Autodesk Fusion 360 part; units mm, degrees
sketch "Sketch1" plane through (0, 0, 0) normal (0, 0, 1) x (1, 0, 0)
  circle A0 centre (0, 0) radius 15 construction
  circle A1 centre (0, 15) radius 1.7
  circle A2 centre (-15, 0) radius 1.7
  circle A3 centre (0, -15) radius 1.7
  circle A4 centre (15, 0) radius 1.7
  circle A5 centre (0, 0) radius 25
  circle A6 centre (0, 25) radius 1.5 construction
  circle A7 centre (-25, 0) radius 1.5 construction
  circle A8 centre (0, -25) radius 1.5 construction
  circle A9 centre (25, 0) radius 1.5 construction
  circle A10 centre (0, 0) radius 31.5
  circle A11 centre (0, 0) radius 25 construction
  dimension "d426" = 30
  dimension "d427" = 3.4
  dimension "d429" = 360
  dimension "d430" = 50
  dimension "d432" = 3
  dimension "d442" = 63
  dimension "d443" = 50
extrude "Extrude1" add sketch "Sketch1" along normal blind 8 contours A5 | A10
hole "Hole2" at (15, 0, 0) at (0, -15, 0) at (-15, 0, 0) at (0, 15, 0) direction (0, 0, -1) diameter 3.4 depth 9 tip angle 118 counterbore diameter 6.5 counterbore depth 3
sketch "Sketch2" plane through (0, 0, 8) normal (0, 0, 1) x (-1, 0, 0)
  circle A0 centre (-15, 0) radius 1.7
  circle A1 centre (15, 0) radius 1.7
  circle A2 centre (0, 15) radius 1.7
  circle A3 centre (0, -15) radius 1.7
  circle A4 centre (0, 0) radius 31.5
  circle A5 centre (0, 0) radius 25
  circle A6 centre (0, -25) radius 1.5 construction
  circle A7 centre (25, 0) radius 1.5 construction
  circle A8 centre (0, 25) radius 1.5 construction
  circle A9 centre (-25, 0) radius 1.5 construction
  dimension "d449" = 50
  dimension "d450" = 3
  dimension "d452" = 360
hole "Hole3" at (0, 25, 8) at (25, 0, 8) at (0, -25, 8) at (-25, 0, 8) direction (0, 0, -1) diameter 6.6 depth 9 tip angle 118 counterbore diameter 11 counterbore depth 6
equation "d426 = promjer_utori"
equation "d443 = promjer_silikona"
equation "promjer_prihvata = promjer_silikona - 10 mm"
equation "promjer_silikona = 50 mm"
equation "promjer_utori = promjer_prihvata - 10 mm"
Read the model definition and answer for the solid it produces. Units are mm, in the model's axes. A direction names the side the tool comes from. Round coordinates to 2 decimals unless told otherwise and drop trailing zeros. Write each loop counter-clockwise with the first axis right and the second up, starting at its lowest first coordinate (ties: lowest second). Pieces come first, ordered by that corner, then holes.
1. The part is cut by section D-D, the plane y = 2.5. Determine the outline of the cut face in (x, z).
2. Straight lines are drawn through the part: L1, parallel to Y at x = 0, z = 4.9; L2, parallel to Y at x = -2, z = 7; L3, parallel to Y at x = 27, z = 5.75. For each, find the intervals that lie inside material, in ascending order.
3. Given pin 1 Ø5.5 at (x, y) = (0, 25) entering from -Z; pin 2 Ø4 at (y, z) = (6.5, 4.5) entering from +X; pin 3 Ø8.5 at (x, y) = (0, -25) entering from +Z; pin 4 Ø1 at (x, z) = (3, 5) entering from -Y, each flat-ended and moving along its own axis, determine where each tip first touches the part or whether it passes through.
4. The part is cut by section A-A, the plane z = 1. State how many separate pieces and enclosed holes the cut face has, then the cut area to 3 significant figures.
5. The part is cut by section B-B, the plane y = 23. Determine the outline of the cut face in (x, z), then the cut area to 3 significant figures.
6. Determine the mould class of faces 1 (the face through (0, 0, 0)), 2 (the face through (1.26, 21.95, 0.99)), 3 (the face through (-4.101, -31.232, 3.944)) for opening direction Y: pulls with the +Y half, pulls with the -Y half, needs draft (parallel to the pull), parting line crosses it, or undercut.
7. The part is cut by section C-C, the plane x = -15. Determine the outline of the cut face in (y, z), then the cut area to 3 significant figures.
8. Which of the six approach directions +Z, -Z, +X, -X, +Y, -Y give full straight-line access (tool end or side, diameter ignored) to faces 4 (the face through (4, -25, 2)), 5 (the face through (-0.221, 13.314, 3.944))?
Values:
1. outline: (-31.4, 0) - (-27.15, 0) - (-27.15, 2) - (-29.9, 2) - (-29.9, 8) - (-31.4, 8) - close; (-22.85, 0) - (22.85, 0) - (22.85, 2) - (20.1, 2) - (20.1, 8) - (-20.1, 8) - (-20.1, 2) - (-22.85, 2) - close; (27.15, 0) - (31.4, 0) - (31.4, 8) - (29.9, 8) - (29.9, 2) - (27.15, 2) - close
2. L1: y = -31.5 to -30.5, -19.5 to -16.7, -13.3 to 13.3, 16.7 to 19.5, 30.5 to 31.5
2. L2: y = -31.44 to -30.12, -19.88 to 19.88, 30.12 to 31.44
2. L3: y = -16.22 to -5.12, 5.12 to 16.22
3. pin 1: passes through
3. pin 2: stops at x = 31.18
3. pin 3: stops at z = 2
3. pin 4: stops at y = -31.4
4. separate pieces: 1
4. enclosed holes: 8
4. area: 2,940 mm2
5. outline: (-21.52, 0) - (-2.62, 0) - (-2.62, 2) - (-5.12, 2) - (-5.12, 8) - (-21.52, 8) - close; (2.62, 0) - (21.52, 0) - (21.52, 8) - (5.12, 8) - (5.12, 2) - (2.62, 2) - close
5. area: 272 mm2
6. face 1: needs draft
6. face 2: undercut
6. face 3: parting line crosses it
7. outline: (-27.7, 0) - (-1.7, 0) - (-1.7, 8) - (-27.7, 8) - close; (1.7, 0) - (27.7, 0) - (27.7, 8) - (1.7, 8) - close
7. area: 416 mm2
8. face 4: +Z
8. face 5: +Z, -Z
